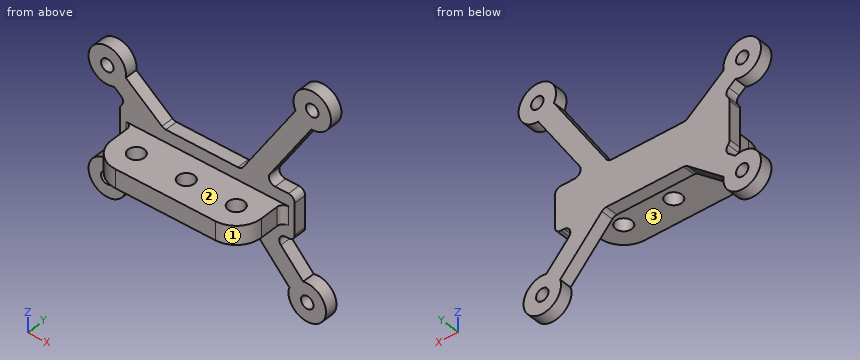
Autodesk Inventor part; units mm, degrees
ref_plane "Work Plane1" through (50.6765, 0, 41.694) normal (0, -1, 0) x (-1, 0, 0)
ref_plane "Work Plane2" through (50.6765, -3.175, 41.694) normal (0, -1, 0) x (-1, 0, 0)
ref_plane "Work Plane7" through (18.0975, -3.175, 36.83) normal (0, 0, 1) x (1, 0, 0)
ref_plane "Work Plane1" through (50.6765, 0, 41.694) normal (0, -1, 0) x (-1, 0, 0)
ref_plane "Work Plane2" through (50.6765, -3.175, 41.694) normal (0, -1, 0) x (-1, 0, 0)
sketch "Sketch2" plane through (50.6765, -3.175, 41.694) normal (0, -1, 0) x (-1, 0, 0)
  circle A0 centre (32.579, -9.106) radius 1.5875 construction
  circle A1 centre (32.579, 18.834) radius 1.5875 construction
  circle A2 centre (-18.221, 23.914) radius 1.5875 construction
  circle A3 centre (-19.491, -24.346) radius 1.5875 construction
  line L0 (-33.461, 26.454) -> (-33.461, -26.886) construction
  line L1 (-33.461, -26.886) -> (30.039, -26.886) construction
  line L2 (30.039, -26.886) -> (32.579, -24.346) construction
  line L3 (32.579, -24.346) -> (32.579, -12.916) construction
  line L4 (32.579, -12.916) -> (35.119, -10.376) construction
  line L5 (35.119, -10.376) -> (35.119, 20.104) construction
  line L6 (35.119, 20.104) -> (32.579, 22.644) construction
  line L7 (32.579, 22.644) -> (32.579, 26.454) construction
  line L8 (32.579, 26.454) -> (-33.461, 26.454) construction
  circle A4 centre (32.579, -9.106) radius 1.5875
  circle A5 centre (-18.221, 23.914) radius 1.5875
  circle A6 centre (32.579, 18.834) radius 1.5875
  circle A7 centre (32.579, -9.106) radius 4.7625
  circle A8 centre (32.579, 18.834) radius 4.7625
  circle A9 centre (-18.221, 23.914) radius 4.7625
  circle A10 centre (-19.491, -24.346) radius 1.5875
  circle A11 centre (-19.491, -24.346) radius 4.7625
  point P0 (50.6765, 41.694)
  dimension "d7" = 9.525
  dimension "d8" = 9.525
  dimension "d9" = 9.525
  dimension "d10" = 3.175
  dimension "d11" = 9.525
extrude "Extrusion2" add sketch "Sketch2" along normal blind 3.175
ref_plane "Work Plane7" through (18.0975, -3.175, 36.83) normal (0, 0, 1) x (1, 0, 0)
ref_plane "Work Plane4" through (18.0975, -3.175, 27.6225) normal (0, 0, 1) x (1, 0, 0)
ref_plane "Work Plane6" through (18.0975, -3.175, 46.0375) normal (0, 0, -1) x (-1, 0, 0)
sketch "Sketch3" plane through (18.0975, -3.175, 36.83) normal (0, 0, 1) x (1, 0, 0)
  line L0 (46.0375, -3.175) -> (55.5625, -3.175) construction
  line L1 (55.5625, 0) -> (46.0375, 0) construction
  line L2 (-4.7625, -3.175) -> (4.7625, -3.175) construction
  line L3 (4.7625, 0) -> (-4.7625, 0) construction
  line L4 (46.0375, -3.175) -> (4.7625, -3.175) construction
  line L5 (4.7625, 0) -> (4.7625, -3.175) construction
  line L6 (25.4, -3.175) -> (25.4, -15.875) construction
  circle A0 centre (25.4, -9.525) radius 2.0574
  circle A1 centre (25.4, -9.525) radius 6.35 construction
  circle A2 centre (12.7, -9.525) radius 2.0574
  arc A3 (6.35, -9.525) -> (12.7, -15.875) centre (12.7, -9.525) ccw
  circle A4 centre (38.1, -9.525) radius 2.0574
  arc A5 (38.1, -15.875) -> (44.45, -9.525) centre (38.1, -9.525) ccw
  line L7 (38.1, -15.875) -> (12.7, -15.875)
  line L8 (44.45, -9.525) -> (44.45, -3.175)
  line L9 (6.35, -9.525) -> (6.35, -3.175)
  line L10 (44.45, -3.175) -> (6.35, -3.175)
  point P0 (-18.0975, 3.175)
  dimension "d14" = 4.1148
  dimension "d15" = 12.7
  dimension "d16" = 4.1148
  dimension "d17" = 12.7
extrude "Extrusion3" add sketch "Sketch3" along normal mid plane 4.7625
sketch "Sketch4" plane through (68.8975, -3.175, 17.78) normal (0, 1, 0) x (1, 0, 0)
  circle A0 centre (1.27, -48.26) radius 4.7625 construction
  circle A1 centre (1.27, -48.26) radius 1.5875 construction
  circle A2 centre (0, 0) radius 1.5875 construction
  circle A3 centre (0, 0) radius 4.7625 construction
  circle A4 centre (-50.8, -5.08) radius 1.5875 construction
  circle A5 centre (-50.8, -5.08) radius 4.7625 construction
  circle A6 centre (-50.8, -33.02) radius 4.7625 construction
  circle A7 centre (-50.8, -33.02) radius 1.5875 construction
  line L0 (-44.45, -16.6687) -> (-6.35, -16.6687) construction
  line L1 (-6.35, -21.4312) -> (-44.45, -21.4312) construction
  line L2 (-44.45, -21.4312) -> (-44.45, -16.6687) construction
  line L3 (-6.35, -21.4312) -> (-6.35, -16.6687) construction
  line L4 (-6.35, -19.05) -> (-44.45, -19.05) construction
  line L5 (-50.8, -33.02) -> (-33.3375, -19.05) construction
  line L6 (-33.3375, -19.05) -> (-50.8, -5.08) construction
  circle A8 centre (0, 0) radius 1.5875 construction
  line L7 (0, 0) -> (-17.4625, -19.05) construction
  circle A9 centre (1.27, -48.26) radius 1.5875 construction
  line L8 (1.27, -48.26) -> (-17.4625, -19.05) construction
  line L9 (-27.4574, -16.6687) -> (-23.3426, -16.6687) construction
  line L10 (-23.3426, -21.4312) -> (-27.4574, -21.4312) construction
  line L11 (-25.4, -21.4312) -> (-25.4, -16.6687) construction
  line L12 (-47.625, -13.4937) -> (-47.625, -24.6062)
  line L13 (-3.175, -24.6062) -> (-3.175, -13.4937)
  line L14 (-2.961, -46.0736) -> (-16.7281, -24.6062)
  line L15 (-15.5996, -13.4937) -> (-4.5423, -1.4313)
  line L16 (-9.1389, -13.4937) -> (-1.0316, -4.6494)
  line L17 (1.048, -43.5027) -> (-11.0704, -24.6062)
  arc A10 (1.048, -43.5027) -> (-2.961, -46.0736) centre (1.27, -48.26) ccw
  arc A11 (-4.5423, -1.4313) -> (-1.0316, -4.6494) centre (0, 0) ccw
  line L18 (-36.471, -24.6062) -> (-46.0918, -32.3029)
  circle A12 centre (-50.8, -33.02) radius 4.7625 construction
  line L19 (-49.0669, -28.584) -> (-44.0947, -24.6062)
  line L20 (-36.471, -13.4937) -> (-46.0918, -5.7971)
  line L21 (-44.0947, -13.4937) -> (-49.0669, -9.516)
  arc A13 (-46.0918, -32.3029) -> (-49.0669, -28.584) centre (-50.8, -33.02) ccw
  arc A14 (-49.0669, -9.516) -> (-46.0918, -5.7971) centre (-50.8, -5.08) ccw
  line L22 (-47.625, -24.6062) -> (-44.0947, -24.6062)
  line L23 (-44.0947, -13.4937) -> (-47.625, -13.4937)
  line L24 (-3.175, -13.4937) -> (-9.1389, -13.4937)
  line L25 (-15.5996, -13.4937) -> (-36.471, -13.4937)
  line L26 (-36.471, -24.6062) -> (-16.7281, -24.6062)
  line L27 (-11.0704, -24.6062) -> (-3.175, -24.6062)
  point P0 (-68.8975, 17.78)
  dimension "d20" = 15.875
  dimension "d21" = 7.9375
  dimension "d28" = 2.3813
  dimension "d29" = 2.3813
  dimension "d30" = 2.3813
  dimension "d31" = 2.3813
  dimension "d32" = 2.3813
  dimension "d33" = 2.3813
  dimension "d34" = 2.3813
  dimension "d35" = 2.3813
  dimension "d36" = 3.175
  dimension "d37" = 3.175
  dimension "d38" = 3.175
  dimension "d39" = 3.175
extrude "Extrusion4" add sketch "Sketch4" against normal up to surface (3.175 mm away)
fillet "Fillet1" radius 1.5875 12 edges at (24.8028, -4.7625, 42.3862) (24.8028, -4.7625, 31.2737) (53.2979, -4.7625, 31.2737) (52.1694, -4.7625, 42.3862) (32.4265, -4.7625, 31.2737) (57.8271, -4.7625, 42.3862) (32.4265, -4.7625, 42.3862) (59.7586, -4.7625, 31.2737) (65.7225, -4.7625, 31.2737) (65.7225, -4.7625, 42.3862) (21.2725, -4.7625, 31.2737) (21.2725, -4.7625, 42.3862)
fillet "Fillet2" radius 1.5875 2 edges at (24.4475, -6.35, 36.83) (62.5475, -6.35, 36.83)
ref_plane "Work Plane3" through (20.6375, 0, 68.58) normal (0, 0, 1) x (1, 0, 0)
ref_plane "Work Plane5" through (84.1375, 0, 15.24) normal (0, 0, -1) x (-1, 0, 0)
properties part number "ChassisPrototypeA4"
Input: part model. Units: mm. Frame: model coordinates. Face numbers are marked on the shaded views. A direction names the side the tool comes from. Round coordinates to 2 decimals unless told otherwise and drop trailing zeros. Write each loop counter-clockwise with the first axis right and the second up, starting at its lowest first coordinate (ties: lowest second). Pieces come first, ordered by that corner, then holes. Notation, with made-up numbers: (81, -29) -> (95, -29) arc R28 ccw to (95, 6) -> close; hole circle Ø6 at (11.5, 74.5). An arc over 180 degrees is marked (long way). Answer as CSV lines item,"result".
1. Contact query for flat-ended pins moving along their axis: P1, Ø3.5, axis at y = -4.5, z = 35.5, coming from the +X side; P2, Ø10, axis at x = 68, z = 44.5, coming from the -Y side; P3, Ø4.5, axis at x = 56.2, y = -12.7, coming from the +Z side. Output: stop coordinate, or through.
Geometry says:
P1,"stops at x = 65.72"
P2,"stops at y = -6.35"
P3,"stops at z = 39.21"
2. Section A-A (z = 66.04). Return the cut outline in (x, y) (3 decimals).
Geometry says:
outline,"(65.405, -6.35) -> (68.58, -6.35) -> (68.58, -3.175) -> (65.405, -3.175) -> close; (71.755, -6.35) -> (74.93, -6.35) -> (74.93, -3.175) -> (71.755, -3.175) -> close"
3. Reachability of the marked faces 1, 2 and 3 from +Z, -Z, +X, -X, +Y, -Y: full face, straight path, thin tool, end or side. Return the list, or none.
Geometry says:
face 1,"+Z, -Z, +X, -Y"
face 2,"+Z, +X, -X, -Y"
face 3,"-Z, +X, -X, -Y"
4. Section D-D (z = 50.8). Return the cut outline in (x, y) (3 decimals).
Geometry says:
outline,"(13.335, -6.35) -> (16.51, -6.35) -> (16.51, -3.175) -> (13.335, -3.175) -> close; (19.685, -6.35) -> (22.86, -6.35) -> (22.86, -3.175) -> (19.685, -3.175) -> close; (57.565, -6.35) -> (63.223, -6.35) -> (63.223, -3.175) -> (57.565, -3.175) -> close"
5. Ray query, L1, parallel to X at y = -5.05, z = 66.04 (3 decimals); L2, parallel to X at y = -5.05, z = 22.86 (3 decimals); L3, parallel to X at y = -5.4, z = 50.8 (3 decimals). Return the intervals inside material, ascending. Write a range as [from, to].
Geometry says:
L1,"x = [65.405, 68.58], [71.755, 74.93]"
L2,"x = [13.335, 16.51], [19.685, 22.86], [61.011, 67.471]"
L3,"x = [13.335, 16.51], [19.685, 22.86], [57.565, 63.223]"
6. Section C-C (y = -11.5). Return the cut outline in (x, z), plus the area to 3 significant figures.
Geometry says:
outline,"(24.45, 34.45) -> (29.13, 34.45) -> (29.13, 39.21) -> (24.45, 39.21) -> close; (32.47, 34.45) -> (41.83, 34.45) -> (41.83, 39.21) -> (32.47, 39.21) -> close; (45.17, 34.45) -> (54.53, 34.45) -> (54.53, 39.21) -> (45.17, 39.21) -> close; (57.87, 34.45) -> (62.55, 34.45) -> (62.55, 39.21) -> (57.87, 39.21) -> close"
area,"134 mm^2"
7. Section B-B (x = 40). Return the cut outline in (y, z) (3 decimals).
Geometry says:
outline,"(-19.05, 34.449) -> (-6.35, 34.449) -> (-6.35, 31.274) -> (-3.175, 31.274) -> (-3.175, 42.386) -> (-6.35, 42.386) -> (-6.35, 39.211) -> (-19.05, 39.211) -> close"
